from build123d import *

# Parameters (mm, degrees)
SKETCH3_R           = 10
BOSS_EXTRUDE1_DEPTH = 25
SKETCH4_W           = 2.5
SKETCH4_H           = 8
BOSS_EXTRUDE2_DEPTH = 30
CUT_EXTRUDE1_REACH  = 37.108
SKETCH5_R           = 2.6
SKETCH6_W           = 5.5
SKETCH6_H           = 21
CUT_EXTRUDE2_DEPTH  = 1.5
SKETCH7_W           = 17
SKETCH7_H           = 7
CUT_EXTRUDE3_DEPTH  = 6
SKETCH8_W           = 2
SKETCH8_H           = 7
CUT_EXTRUDE4_DEPTH  = 4
BOSS_EXTRUDE3_DEPTH = 1.5
CUT_EXTRUDE5_REACH  = 35.166


with BuildPart() as part:
    # Sketch3 → Boss-Extrude1 (new body)
    with BuildSketch(Plane(origin=(0, 0, 0), x_dir=(1, 0, 0), z_dir=(0, 1, 0))):
        with Locations(Location((0, 0, 0), (0, 0, 270))):
            Circle(SKETCH3_R)
    extrude(amount=BOSS_EXTRUDE1_DEPTH)

    # Sketch4 → Boss-Extrude2 (add)
    with BuildSketch(Plane(origin=(0, 0, 0), x_dir=(-1, 0, 0), z_dir=(0, -1, 0))):
        with Locations((-4, 0)):
            Rectangle(SKETCH4_W, SKETCH4_H)
    extrude(amount=BOSS_EXTRUDE2_DEPTH)

    # Sketch5 → Cut-Extrude1 (cut, up to next)
    with BuildSketch(Plane(origin=(5.25, 0, 0), x_dir=(0, 0, -1), z_dir=(1, 0, 0)), mode=Mode.PRIVATE) as cut_extrude1_sk1:
        with Locations((0, -18.4)):
            Circle(SKETCH5_R)
    cut_extrude1_tool1 = extrude(cut_extrude1_sk1.sketch, amount=-CUT_EXTRUDE1_REACH, mode=Mode.PRIVATE) & part.part
    add(cut_extrude1_tool1.solids().sort_by_distance((5.25, -18.4, 0))[0], mode=Mode.SUBTRACT)

    # Sketch6 → Cut-Extrude2 (cut)
    with BuildSketch(Plane.ZY.offset(-2.75)):
        with Locations((0, -18.4)):
            Rectangle(SKETCH6_W, SKETCH6_H)
    extrude(amount=-CUT_EXTRUDE2_DEPTH, mode=Mode.SUBTRACT)

    # Sketch7 → Cut-Extrude3 (cut)
    with BuildSketch(Plane(origin=(0, 25, 0), x_dir=(1, 0, 0), z_dir=(0, 1, 0))):
        Rectangle(SKETCH7_W, SKETCH7_H)
    extrude(amount=-CUT_EXTRUDE3_DEPTH, mode=Mode.SUBTRACT)

    # Sketch8 → Cut-Extrude4 (cut)
    with BuildSketch(Plane(origin=(0, 19, 0), x_dir=(1, 0, 0), z_dir=(0, 1, 0))):
        with Locations((-2.25, 0)):
            Rectangle(SKETCH8_W, SKETCH8_H)
    extrude(amount=-CUT_EXTRUDE4_DEPTH, mode=Mode.SUBTRACT)

    # Sketch9 → Boss-Extrude3 (add)
    with BuildSketch(Plane.ZY.offset(-4.25)):
        Polygon((-2.75, -28.9), (-2.75, -21.9), (-1.5, -28.9), align=None)
        Polygon((1.5, -28.9), (2.75, -28.9), (2.75, -21.9), align=None)
        Polygon((2.75, -7.9), (2.75, -14.9), (1.5, -7.9), align=None)
        Polygon((-1.5, -7.9), (-2.75, -7.9), (-2.75, -14.9), align=None)
    extrude(amount=BOSS_EXTRUDE3_DEPTH)

    # Sketch11 → Cut-Extrude5 (cut, up to next)
    with BuildSketch(Plane(origin=(0, 0, 0), x_dir=(-1, 0, 0), z_dir=(0, -1, 0)), mode=Mode.PRIVATE) as cut_extrude5_sk1:
        with BuildLine():
            Line((8.511022265, 5.25), (-8.511022265, 5.25))
            ThreePointArc((-8.511022265, 5.25), (0, 10), (8.511022265, 5.25))
        make_face()
    cut_extrude5_tool1 = extrude(cut_extrude5_sk1.sketch, amount=-CUT_EXTRUDE5_REACH, mode=Mode.PRIVATE) & part.part
    # Sketch11 → Cut-Extrude5 (cut, up to next)
    with BuildSketch(Plane(origin=(0, 0, 0), x_dir=(-1, 0, 0), z_dir=(0, -1, 0)), mode=Mode.PRIVATE) as cut_extrude5_sk2:
        with BuildLine():
            Line((8.511022265, -5.25), (-8.511022265, -5.25))
            ThreePointArc((-8.511022265, -5.25), (0, -10), (8.511022265, -5.25))
        make_face()
    cut_extrude5_tool2 = extrude(cut_extrude5_sk2.sketch, amount=-CUT_EXTRUDE5_REACH, mode=Mode.PRIVATE) & part.part
    add(cut_extrude5_tool1.solids().sort_by_distance((0, 0, -7.194917))[0], mode=Mode.SUBTRACT)
    add(cut_extrude5_tool2.solids().sort_by_distance((0, 0, 7.194917))[0], mode=Mode.SUBTRACT)


solid = part.part
Can you work these out from the model? Positions are in its coordinate system, mm. A direction names the side the tool comes from. Coordinates: 2 decimals unless noted, no trailing zeros. Write each loop counter-clockwise with the first axis right and the second up, starting at its lowest first coordinate (ties: lowest second). Pieces come first, ordered by that corner, then holes.
Q1. Imagine slicing it at B-B, the plane z = 0. List the corners of the cut face in (x, y) for me.
Results found:
outline: (-10, 0) - (2.75, 0) - (2.75, -7.9) - (4.25, -7.9) - (4.25, -15.8) - (5.25, -15.8) - (5.25, 0) - (10, 0) - (10, 25) - (8.5, 25) - (8.5, 19) - (-1.25, 19) - (-1.25, 15) - (-3.25, 15) - (-3.25, 19) - (-8.5, 19) - (-8.5, 25) - (-10, 25) - close; (2.75, -30) - (5.25, -30) - (5.25, -21) - (4.25, -21) - (4.25, -28.9) - (2.75, -28.9) - close
Q2. For P1, Ø1.8, axis at y = 21.5, z = -1, coming from the -X side; P2, Ø3, axis at x = 4.5, z = -1, coming from the +Y side; P3, Ø1.2, axis at x = 4.5, y = -10, coming from the -Z side; P4, Ø1, axis at y = -20, z = 3.5, coming from the +X side, each with a flat end and sliding along its axis, tell me the tip position at first contact or that it passes through.
Results found:
P1: stops at x = -10
P2: stops at y = 19
P3: stops at z = -4
P4: stops at x = 5.25
Q3. Imagine slicing it at C-C, the plane x = -0.75. List the corners of the cut face in (y, z) for me.
Results found:
outline: (0, -5.25) - (25, -5.25) - (25, -3.5) - (19, -3.5) - (19, 3.5) - (25, 3.5) - (25, 5.25) - (0, 5.25) - close
Q4. Imagine slicing it at D-D, the plane y = 3. List the corners of the cut face in (x, z) for me, plus the area to 3 significant figures.
Results found:
outline: (-8.51, -5.25) - (8.51, -5.25) arc R10 ccw to (8.51, 5.25) - (-8.51, 5.25) arc R10 ccw to start
area: 200 mm2
Q5. Which directions (+Z, -Z, +X, -X, +Y, -Y) give clear straight access to the entire face, cutting with the end or side of a thin tool? Please do faces 4 (the face through (3.51, -11.449, -2.134)), 5 (the face through (0, 12, -5.25)), 6 (the face through (-3.25, 17, 0)).
Results found:
face 4: -X
face 5: -Z, +X, -X, +Y, -Y
face 6: +Y
Q6. If we mould it in two halves opening along X, with no side actions, what happens to faces 1 (the face through (2.75, -11, 3)), 2 (the face through (3, -28.9, 0)), 3 (the face through (-8.5, 22, 0))? For each: +X half, -X half, draft (parallel to the pull), parting line (faces both ways), or undercut.
Results found:
face 1: -X half
face 2: draft
face 3: undercut
Q7. Imagine slicing it at A-A, the plane y = -18.4. List the corners of the cut face in (x, z) for me, plus the area to 3 significant figures.
Results found:
outline: (2.75, -4) - (5.25, -4) - (5.25, -2.6) - (4.25, -2.6) - (4.25, -2.75) - (2.75, -2.75) - close; (2.75, 2.75) - (4.25, 2.75) - (4.25, 2.6) - (5.25, 2.6) - (5.25, 4) - (2.75, 4) - close
area: 6.55 mm2
Q8. Please list where these lines run through material, in increasing order: L1, parallel to Y at x = 5, z = 0; L2, parallel to X at y = 16, z = 0; L3, parallel to X at y = -28, z = 2.5.
Results found:
L1: y = -30 to -21, -15.8 to 19
L2: x = -10 to -3.25, -1.25 to 10
L3: x = 2.75 to 5.25
